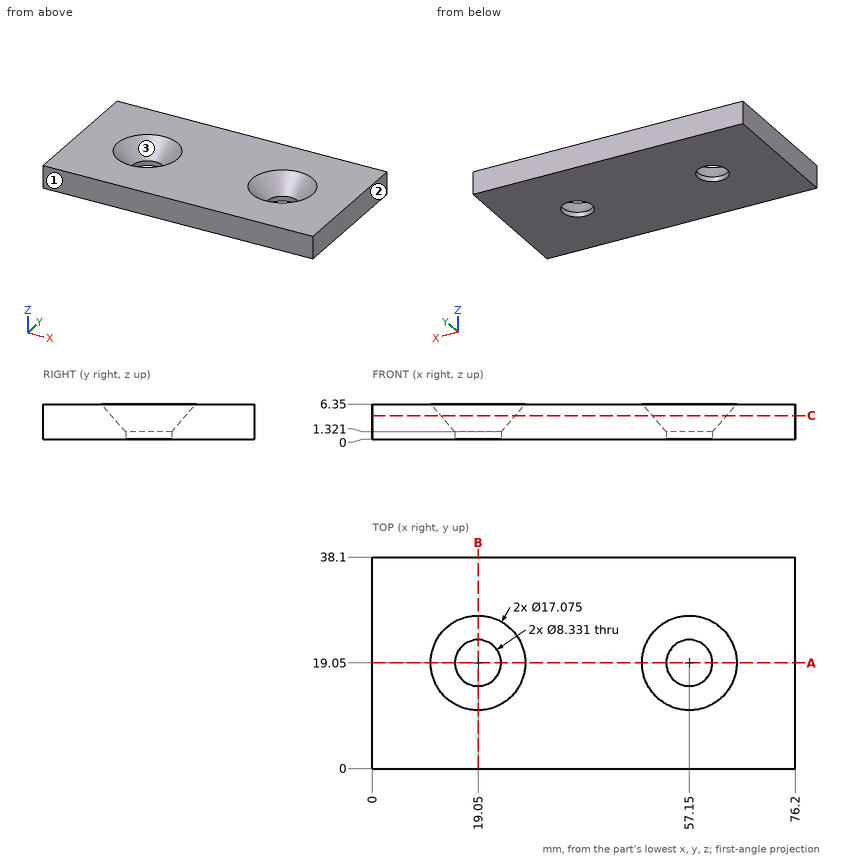
The drawing under review shows one solid part. Ordinate dimensions are in mm from its lowest x, y, z. Give positions to 0.01 mm unless a question says otherwise; leave off trailing zeros. Loops run counter-clockwise (first coordinate to the right, second up) from the corner with the lowest first, then second, coordinate; pieces in that order, holes last. Notation, with made-up numbers: M 33,78.25 L 92,78.25 A26 ccw 92,110.25 Z; hole C 42,88.5 d1. An arc over 180 degrees is marked long. One line per question, with ' | ' between items. Start each with the question number.
1. Insertion check: P1, Ø5, axis at x = 19.05, y = 19.05, coming from the -Z side (3 decimals). The pin has a flat end and moves straight along its axis. Give the tip position at first contact, or say it passes through.
2. To check wall thickness, follow L1, parallel to Y at x = 57.15, z = 0.8; L2, parallel to X at y = 22, z = 2; L3, parallel to X at y = 13.5, z = 4.5. State the ranges of each line that lie inside material, in increasing order.
3. Add section A-A (y = 19.05). Write out the cut boundary in (x, z), plus the area to 3 significant figures.
4. Add section C-C (z = 4.25). Write out the cut boundary in (x, y).
5. Add section B-B (x = 19.05). Write out the cut boundary in (y, z), plus the area to 3 significant figures.
6. The part is to be moulded in two halves that separate along Y. For the marked faces 1, 2 and 3, say which applies: released by +Y, released by -Y, zero draft, split by the parting line, or undercut.
Worked out:
1) P1: passes through
2) L1: y = 0 to 14.88, 23.22 to 38.1 | L2: x = 0 to 15.32, 22.78 to 53.42, 60.88 to 76.2 | L3: x = 0 to 14.9, 23.2 to 53, 61.3 to 76.2
3) outline: M 0,0 L 14.88,0 L 14.88,1.32 L 10.51,6.35 L 0,6.35 Z; M 23.22,0 L 52.98,0 L 52.98,1.32 L 48.61,6.35 L 27.59,6.35 L 23.22,1.32 Z; M 61.32,0 L 76.2,0 L 76.2,6.35 L 65.69,6.35 L 61.32,1.32 Z | area: 334 mm²
4) outline: M 0,0 L 76.2,0 L 76.2,38.1 L 0,38.1 Z; hole C 19.05,19.05 d13.42; hole C 57.15,19.05 d13.42
5) outline: M 0,0 L 14.88,0 L 14.88,1.32 L 10.51,6.35 L 0,6.35 Z; M 23.22,0 L 38.1,0 L 38.1,6.35 L 27.59,6.35 L 23.22,1.32 Z | area: 167 mm²
6) face 1: released by -Y | face 2: zero draft | face 3: undercut
